Read the model definition and answer for the solid it produces. Units are mm, in the model's axes. A direction names the side the tool comes from. Coordinates: 2 decimals unless noted, no trailing zeros. Loops run counter-clockwise (first coordinate to the right, second up) from the corner with the lowest first, then second, coordinate; pieces in that order, holes last. Notation, with made-up numbers: M 59.25,49 L 65.25,49 A6 cw 65.25,55 Z; hole C 4.5,30.25 d4. An arc over 180 degrees is marked long. Put each result on its own line as item: value.
from build123d import *

# Parameters (mm, degrees)
F0_W      = 101.6
F0_H      = 38.1
F1_DEPTH  = 38.1
F2_W      = 91.44
F2_H      = 27.94
F3_DEPTH  = 20.32
F4_R      = 5.08
F5_DEPTH  = 38.101
F6_W      = 22.86
F6_H      = 5.08
F7_DEPTH  = 1.27
F8_W      = 12.7
F8_H      = 5.08
F9_DEPTH  = 12.7
F10_R     = 1.905
F11_DEPTH = 10.161


with BuildPart() as f1:
    # F0 (on Front) → F1 (new body)
    with BuildSketch(Plane.XZ):
        with Locations((-2.376233, -0.464275)):
            Rectangle(F0_W, F0_H)
    extrude(amount=F1_DEPTH)

    # F2 (on face) → F3 (cut)
    with BuildSketch(Plane.XY.offset(18.585725)):
        with Locations((-2.376233, -19.05)):
            Rectangle(F2_W, F2_H)
    extrude(amount=-F3_DEPTH, mode=Mode.SUBTRACT)

    # F4 (on face) → F5 (cut, through all)
    with BuildSketch(Plane.XZ.offset(38.1)):
        with Locations((-27.776233, -11.894275)):
            Circle(F4_R)
        with Locations((23.023767, -11.894275)):
            Circle(F4_R)
    extrude(amount=-F5_DEPTH, mode=Mode.SUBTRACT)

    # F6 (on face) → F7 (join)
    with BuildSketch(Plane(origin=(-53.176233, 0, 0), x_dir=(0, -1, 0), z_dir=(-1, 0, 0))):
        with Locations((19.05, 12.235725)):
            Rectangle(F6_W, F6_H)
        with Locations((19.05, 3.769143)):
            Rectangle(F6_W, F6_H)
        with Locations((19.05, -4.689057)):
            Rectangle(F6_W, F6_H)
    extrude(amount=F7_DEPTH)

    # F8 (on face) → F9 (join)
    with BuildSketch(Plane(origin=(-53.176233, 0, 0), x_dir=(0, -1, 0), z_dir=(-1, 0, 0))):
        with Locations((19.05, -11.894275)):
            Rectangle(F8_W, F8_H)
    extrude(amount=F9_DEPTH)

    # F10 (on face) → F11 (cut, through all)
    with BuildSketch(Plane.XY.offset(-9.354275)):
        with Locations((-56.986233, -19.05)):
            Circle(F10_R)
    extrude(amount=-F11_DEPTH, mode=Mode.SUBTRACT)


solid = f1.part
1) Find section D-D, the plane z = 7.5. Write down the section's boundary in (x, y).
Answer list:
outline: M -53.18,-38.1 L 48.42,-38.1 L 48.42,0 L -53.18,0 Z; hole M -48.1,-33.02 L 43.34,-33.02 L 43.34,-5.08 L -48.1,-5.08 Z
2) Find section A-A, the plane z = 12. Write down the section's boundary in (x, y), plus the area to 3 significant figures.
Answer list:
outline: M -54.45,-30.48 L -53.18,-30.48 L -53.18,-38.1 L 48.42,-38.1 L 48.42,0 L -53.18,0 L -53.18,-7.62 L -54.45,-7.62 Z; hole M -48.1,-33.02 L 43.34,-33.02 L 43.34,-5.08 L -48.1,-5.08 Z
area: 1,350 mm^2
3) Straight lines are drawn through the part: line 1 (X direction, y = -19, z = -12); line 2 (Z direction, x = -54, y = -21); line 3 (Y direction, x = -46.5, z = 2.5). For each, find the intervals that lie inside material, in ascending order. Write a range as [from, to].
Answer list:
line 1: x = [-65.88, -58.89], [-55.08, -32.86], [-22.7, 17.94], [28.1, 48.42]
line 2: z = [-14.43, -9.35], [-7.23, -2.15], [1.23, 6.31], [9.7, 14.78]
line 3: y = [-38.1, -33.02], [-5.08, 0]
4) Find section C-C, the plane x = 0. Write down the section's boundary in (y, z).
Answer list:
outline: M -38.1,-19.51 L 0,-19.51 L 0,18.59 L -5.08,18.59 L -5.08,-1.73 L -33.02,-1.73 L -33.02,18.59 L -38.1,18.59 Z
5) Find section B-B, the plane y = -19.05. Count the separate pieces of the cut face and the enclosed holes in it, plus the area to 3 significant figures.
Answer list:
separate pieces: 2
enclosed holes: 2
area: 1,920 mm^2
6) Which of the six approach directions +Z, -Z, +X, -X, +Y, -Y give full straight-line access (tool end or side, diameter ignored) to faces 4 (the flat face through (-59.4, -19, -9.354)), 5 (the flat face through (43.344, -19, 9)), 6 (the flat face through (-59.4, -19, -14.434)), 7 (the flat face through (-54.446, -19, 4))?
Answer list:
face 4: -X, +Y, -Y
face 5: +Z
face 6: -Z, -X, +Y, -Y
face 7: +Z, -X, +Y, -Y
7) Determine the mould class of faces 1 (the flat face through (-2.6, -4.8, 18.586)), 2 (the flat face through (-54.446, -19, -5)), 3 (the cylindrical face through (17.95, -19.32, -11.67)) for opening direction Z: released by +Z, released by -Z, zero draft, split by the parting line, or undercut.
Answer list:
face 1: released by +Z
face 2: zero draft
face 3: undercut
8) Given pin 1 Ø14 at (x, y) = (-14, -18.5) entering from +Z; pin 2 Ø1.4 at (x, y) = (-54, -15.5) entering from +Z; pin 3 Ø1 at (x, z) = (-54, 3.5) entering from -Y, each flat-ended and moving along its own axis, determine where each tip first touches the part or whether it passes through.
Answer list:
pin 1: stops at z = -1.73
pin 2: stops at z = 14.78
pin 3: stops at y = -30.48
